from build123d import *

# Parameters (mm, degrees)
EXTRUDE001_DEPTH = 2
EXTRUDE002_DEPTH = 6
EXTRUDE_DEPTH    = 1
CHAMFER_SIZE     = 0.8


with BuildPart() as extrude001:
    # Sketch001 → Extrude001 (new body)
    with BuildSketch(Plane.XY):
        Polygon((-4.5, 4.2), (4.5, 4.2), (4.5, 2.6), (2.9, 1), (-2.9, 1), (-4.5, 2.6), align=None)
    extrude(amount=EXTRUDE001_DEPTH)


with BuildPart() as extrude002:
    # Sketch002 → Extrude002 (new body)
    with BuildSketch(Plane.XY):
        Polygon((-3.5, 3.6), (-2, 3.6), (-2, 2.6), (2, 2.6), (2, 3.6), (3.5, 3.6), (3.5, 2.6), (2.5, 1.6), (-2.5, 1.6), (-3.5, 2.6), align=None)
    extrude(amount=EXTRUDE002_DEPTH)


with BuildPart() as chamfer_body:
    # Sketch → Extrude (new body)
    with BuildSketch(Plane.XY):
        Polygon((-5.5, 5.2), (5.5, 5.2), (5.5, 2.6), (2.9, 0), (-2.9, 0), (-5.5, 2.6), align=None)
    extrude(amount=EXTRUDE_DEPTH)

    # Fusion: union Extrude001, Extrude002
    add(extrude001.part)
    add(extrude002.part)

    # Chamfer
    chamfer_edges = [chamfer_body.edges().sort_by_distance(p)[0] for p in [
        (0, 5.2, 0),
        (-5.5, 3.9, 0),
        (5.5, 3.9, 0),
        (-4.2, 1.3, 0),
        (4.2, 1.3, 0),
        (0, 0, 0),
    ]]
    chamfer(chamfer_edges, length=CHAMFER_SIZE)


solid = chamfer_body.part
For this review, take the finished solid that the model builds, in its own axes (mm). A direction names the side the tool comes from. Round coordinates to 2 decimals unless told otherwise and drop trailing zeros. Loops run counter-clockwise (first coordinate to the right, second up) from the corner with the lowest first, then second, coordinate; pieces in that order, holes last. Notation, with made-up numbers: (-4, 50.5) - (30, 50.5) arc R19 cw to (30, 87.5) - close; hole circle Ø8 at (73, 7). An arc over 180 degrees is marked (long way). One line per item, written item: value. Start each with the question number.
Item 1: For L1, parallel to X at y = 3.3, z = 2.4; L2, parallel to Y at x = 0.5, z = 1.1; L3, parallel to Z at x = -3, y = 1.3, list the stretches that pass through material, from the lowest coordinate up.
Item 2: Take a section at B-B (z = 1.5). Give the boundary of the cut face in (x, y).
Item 3: Take a section at D-D (z = 3.4). Give the boundary of the cut face in (x, y).
Item 4: The part is to be moulded in two halves that separate along X. For faces 1 (the flat face through (-3.5, 3, 4)), 2 (the flat face through (0, 3, 0)), 3 (the flat face through (-2, 3, 4)), say which applies: +X half, -X half, draft (parallel to the pull), parting line (faces both ways), or undercut.
Item 5: For faces 4 (the flat face through (-4.5, 3.4, 1.5)), 5 (the flat face through (0, 1.6, 4)), 6 (the flat face through (-3, 3.6, 4)), 7 (the flat face through (4.5, 3.4, 1.5)), list the 3-axis set-ups (+Z, -Z, +X, -X, +Y, -Y) from which the entire face can be reached by the end or side of a thin tool; tool diameter is ignored.
Item 6: Take a section at A-A (x = 1). Give the boundary of the cut face in (y, z), plus the area to 3 significant figures.
Item 7: Take a section at C-C (y = 1.4). Give the boundary of the cut face in (x, z).
Item 8: Clearance check with flat-ended pins moving along their axes: pin 1 Ø0.5 at (y, z) = (3.5, 4) entering from -X; pin 2 Ø0.5 at (x, z) = (1.5, 1.5) entering from +Y; pin 3 Ø3 at (x, z) = (-0.5, 4.5) entering from -Y. State where each tip first meets the part, or that it passes through.
Answer below:
1. L1: x = -3.5 to -2, 2 to 3.5
1. L2: y = 1 to 4.2
1. L3: z = 0 to 2
2. outline: (-4.5, 2.6) - (-2.9, 1) - (2.9, 1) - (4.5, 2.6) - (4.5, 4.2) - (-4.5, 4.2) - close
3. outline: (-3.5, 2.6) - (-2.5, 1.6) - (2.5, 1.6) - (3.5, 2.6) - (3.5, 3.6) - (2, 3.6) - (2, 2.6) - (-2, 2.6) - (-2, 3.6) - (-3.5, 3.6) - close
4. face 1: -X half
4. face 2: draft
4. face 3: undercut
5. face 4: +Z, -X, +Y, -Y
5. face 5: +Z, +X, -X, -Y
5. face 6: +Z, +X, -X, +Y
5. face 7: +Z, +X, +Y, -Y
6. outline: (0, 0.8) - (0.8, 0) - (4.4, 0) - (5.2, 0.8) - (5.2, 1) - (4.2, 1) - (4.2, 2) - (2.6, 2) - (2.6, 6) - (1.6, 6) - (1.6, 2) - (1, 2) - (1, 1) - (0, 1) - close
6. area: 11.8 mm2
7. outline: (-4.3, 0.8) - (-3.17, 0) - (3.17, 0) - (4.3, 0.8) - (4.3, 1) - (3.3, 1) - (3.3, 2) - (-3.3, 2) - (-3.3, 1) - (-4.3, 1) - close
8. pin 1: stops at x = -3.5
8. pin 2: stops at y = 4.2
8. pin 3: stops at y = 1.6
